from build123d import *

# Parameters (mm, degrees)
F1_DEPTH = 1.588
F2_R     = 2.5
F3_DEPTH = 1.589


with BuildPart() as f1:
    # F0 (on Top) → F1 (new body)
    with BuildSketch(Plane.XY):
        Polygon((33.02, 26.67), (-33.02, 26.67), (-33.02, -26.67), (33.02, -26.67), (33.02, -24.003), (33.02, 14.097), align=None)
        Polygon((35.56, 11.557), (33.02, 14.097), (33.02, -24.003), (35.56, -21.463), align=None)
    extrude(amount=F1_DEPTH)

    # F2 (on face) → F3 (cut, through all)
    with BuildSketch(Plane.XY.offset(1.588)):
        with Locations((-18.220948, 22.122128)):
            Circle(F2_R)
        with Locations((31.972159, 9.393649)):
            Circle(F2_R)
        with Locations((31.171337, -19.547544)):
            Circle(F2_R)
        with Locations((-21.635612, -21.463)):
            Circle(F2_R)
    extrude(amount=-F3_DEPTH, mode=Mode.SUBTRACT)


solid = f1.part
Verification items for the finished model (mm, model axes). A direction names the side the tool comes from. Give positions to 0.01 mm unless a question says otherwise; leave off trailing zeros. Loops run counter-clockwise (first coordinate to the right, second up) from the corner with the lowest first, then second, coordinate; pieces in that order, holes last.
1) Sectioned sample at A-A, the plane x = -22.5. Enter the section's corners in (y, z).
2) Thickness scan on line 1 along Y through (x, z) = (30, 1); line 2 along X through (y, z) = (20, 0.75); line 3 along X through (y, z) = (23.5, 0.3). Record the ranges inside material, lowest first.
3) Depth check by flat-ended pin: pin 1 Ø0.5 at (y, z) = (-25.5, 0.5) entering from +X; pin 2 Ø3 at (x, y) = (31.17, -19.55) entering from -Z. Enter the tip coordinate at first touch or a pass-through.
4) Set-up check for faces 1 (the flat face through (-33.02, 0, 1)), 2 (the flat face through (33.02, 20, 1)), 3 (the flat face through (33.02, -25, 1)): record each of +Z, -Z, +X, -X, +Y, -Y from which the full face is reachable in a straight line by a thin tool's end or side.
5) Draft check along X on faces 4 (the cylindrical face through (33.556, -18.797, 0.805)), 5 (the flat face through (34.308, 12.809, 0.783)), 6 (the flat face through (1, 0, 0)). Enter one of: pulls with the +X half, pulls with the -X half, needs draft (parallel to the pull), parting line crosses it, or undercut.
6) Sectioned sample at B-B, the plane z = 0.75. Enter the section's corners in (x, y).
Answers:
1. outline: (-26.67, 0) - (-23.81, 0) - (-23.81, 1.59) - (-26.67, 1.59) - close; (-19.12, 0) - (26.67, 0) - (26.67, 1.59) - (-19.12, 1.59) - close
2. line 1: y = -26.67 to -21.76, -17.34 to 7.86, 10.93 to 26.67
2. line 2: x = -33.02 to -19.54, -16.9 to 33.02
2. line 3: x = -33.02 to -20.31, -16.13 to 33.02
3. pin 1: stops at x = 33.02
3. pin 2: passes through
4. face 1: +Z, -Z, -X, +Y, -Y
4. face 2: +Z, -Z, +X, +Y
4. face 3: +Z, -Z, +X, -Y
5. face 4: undercut
5. face 5: pulls with the +X half
5. face 6: needs draft
6. outline: (-33.02, -26.67) - (33.02, -26.67) - (33.02, -24) - (35.56, -21.46) - (35.56, 11.56) - (33.02, 14.1) - (33.02, 26.67) - (-33.02, 26.67) - close; hole circle Ø5 at (-21.64, -21.46); hole circle Ø5 at (-18.22, 22.12); hole circle Ø5 at (31.17, -19.55); hole circle Ø5 at (31.97, 9.39)
